Design review of the part built by this model. Coordinates are the model's own, in mm. A direction names the side the tool comes from. Give positions to 0.01 mm unless a question says otherwise; leave off trailing zeros. Loops run counter-clockwise (first coordinate to the right, second up) from the corner with the lowest first, then second, coordinate; pieces in that order, holes last. Notation, with made-up numbers: (80.25, -21) - (132.25, -21) arc R11 cw to (132.25, -6) - close; hole circle Ø4 at (21, 88). An arc over 180 degrees is marked (long way). Write each question's results on one line, items separated by ' | '.
from build123d import *

# Parameters (mm, degrees)
SKETCH_1_W          = 3
SKETCH_1_H          = 15
EXTRUDE_1_DEPTH     = 3
SKETCH_2_R          = 1.5
SKETCH_2_R_2        = 2.03
SKETCH_2_R_3        = 3.75
CUT_EXTRUDE_1_DEPTH = 10


with BuildPart() as part:
    # 草图1 → 凸台-拉伸1 (new body)
    with BuildSketch(Plane.XY):
        Polygon((2.5, 3), (0, 3), (0, 117), (2.5, 117), (2.5, 120), (17.5, 120), (17.5, 117), (32.5, 117), (32.5, 120), (47.5, 120), (47.5, 117), (62.5, 117), (62.5, 120), (77.5, 120), (77.5, 117), (80, 117), (80, 3), (77.5, 3), (77.5, 0), (62.5, 0), (62.5, 3), (47.5, 3), (47.5, 0), (32.5, 0), (32.5, 3), (17.5, 3), (17.5, 0), (2.5, 0), align=None)
        with Locations((77, 27.5)):
            Rectangle(SKETCH_1_W, SKETCH_1_H, mode=Mode.SUBTRACT)
        with Locations((3, 27.5)):
            Rectangle(SKETCH_1_W, SKETCH_1_H, mode=Mode.SUBTRACT)
    extrude(amount=EXTRUDE_1_DEPTH)

    # 草图2 → 切除-拉伸1 (cut)
    with BuildSketch(Plane.XY.offset(3)):
        with Locations((31.5, 45)):
            Circle(SKETCH_2_R)
        with Locations((48.5, 45)):
            Circle(SKETCH_2_R)
        with Locations((40, 54)):
            Circle(SKETCH_2_R_2)
        with Locations((40, 65)):
            Circle(SKETCH_2_R_3)
    extrude(amount=-CUT_EXTRUDE_1_DEPTH, mode=Mode.SUBTRACT)


solid = part.part
(1) Draft analysis for pull direction Y (two halves, no side actions). For faces 5 (the flat face through (40, 120, 1)), 6 (the flat face through (77, 20, 1)), 7 (the flat face through (77.5, 119, 1)), state which applies: pulls with the +Y half, pulls with the -Y half, needs draft (parallel to the pull), parting line crosses it, or undercut.
Answers below:
face 5: pulls with the +Y half | face 6: undercut | face 7: needs draft
(2) Take a section at A-A on y = 65. Give the boundary of the cut face in (x, z), plus the area to 4 significant figures.
Answers below:
outline: (0, 0) - (36.25, 0) - (36.25, 3) - (0, 3) - close; (43.75, 0) - (80, 0) - (80, 3) - (43.75, 3) - close | area: 217.5 mm2
(3) Tool access review of faces 1 (the flat face through (70, 0, 1)), 2 (the flat face through (25, 117, 1)), 3 (the flat face through (77, 35, 1)), 4 (the flat face through (62.5, 1, 1)): name each direction out of +Z, -Z, +X, -X, +Y, -Y from which nothing blocks a thin tool from reaching the whole face with its end or side.
Answers below:
face 1: +Z, -Z, +X, -X, -Y | face 2: +Z, -Z, +Y | face 3: +Z, -Z | face 4: +Z, -Z, -Y
(4) Wall thickness on line 1 along X through (y, z) = (21, 0.65); line 2 along Y through (x, z) = (48.5, 2.35); line 3 along Y through (x, z) = (61.5, 0.5): over which ranges is each line inside the solid? List them lowest first. Write a range as from..to.
Answers below:
line 1: 0..1.5, 4.5..75.5, 78.5..80 | line 2: 3..43.5, 46.5..117 | line 3: 3..117
(5) Take a section at C-C on x = 40. Give the boundary of the cut face in (y, z), plus the area to 3 significant figures.
Answers below:
outline: (0, 0) - (51.97, 0) - (51.97, 3) - (0, 3) - close; (56.03, 0) - (61.25, 0) - (61.25, 3) - (56.03, 3) - close; (68.75, 0) - (120, 0) - (120, 3) - (68.75, 3) - close | area: 325 mm2
(6) Insertion check: P1, Ø1.5, axis at x = 25.5, z = 2, coming from the +Y side; P2, Ø0.9, axis at y = 118, z = 1.5, coming from the -X side; P3, Ø1, axis at x = 9, z = 2.5, coming from the -Y side. Each pin has a flat end and moves straight along its axis. Give the tip position at first contact, or say it passes through.
Answers below:
P1: y = 117 | P2: x = 2.5 | P3: y = 0
(7) Take a section at B-B on y = 45. Give the boundary of the cut face in (x, z), plus the area to 3 significant figures.
Answers below:
outline: (0, 0) - (30, 0) - (30, 3) - (0, 3) - close; (33, 0) - (47, 0) - (47, 3) - (33, 3) - close; (50, 0) - (80, 0) - (80, 3) - (50, 3) - close | area: 222 mm2
(8) Take a section at D-D on z = 1.45. Count the separate pieces of the cut face and the enclosed holes in it, plus the area to 3 significant figures.
Answers below:
separate pieces: 1 | enclosed holes: 6 | area: 9,230 mm2
